Read the model definition and answer for the solid it produces. Units are mm, in the model's axes. Face numbers are marked on the shaded views. A direction names the side the tool comes from. Coordinates: 2 decimals unless noted, no trailing zeros. Write each loop counter-clockwise with the first axis right and the second up, starting at its lowest first coordinate (ties: lowest second). Pieces come first, ordered by that corner, then holes. Notation, with made-up numbers: (52, 11.5) -> (95, 11.5) arc R21 ccw to (95, 16.5) -> close; hole circle Ø9 at (33, 50). An arc over 180 degrees is marked (long way). Answer as a JSON object with one key per item and string values. Group by question number.
(1) Find section A-A (y = -11). Give the vertices of the cut face in (x, z).
(2) Straight lines are drawn through the part: L1, parallel to Y at x = 0, z = 14.4; L2, parallel to X at y = 1.65, z = -9.5; L3, parallel to Z at x = -1.75, y = -6.25. For each, find the intervals that lie inside material, in ascending order.
(3) Flat-ended cylindrical pins translate along their axes: P1, Ø4, axis at x = 0, z = -9.5, coming from the -Y side; P2, Ø4, axis at x = 0.5, y = -6, coming from the -Z side. Find the tip coordinate at first contact, or state that the pin passes through.
(4) Find section B-B (x = 0). Give the vertices of the cut face in (y, z).
(5) Which of the six approach directions +Z, -Z, +X, -X, +Y, -Y give full straight-line access (tool end or side, diameter ignored) to the marked faces 1 and 2?
(6) Find section C-C (z = -9.5). Give the vertices of the cut face in (x, y), then the cut area to 3 significant figures.
(7) Find section D-D (y = 0.5). Give the vertices of the cut face in (x, z).
(8) For a pull along Y with two mould halves and no side action, classify the marked faces 3, 4 and 5 as +Y half, -Y half, draft (parallel to the pull), parting line (faces both ways), or undercut.
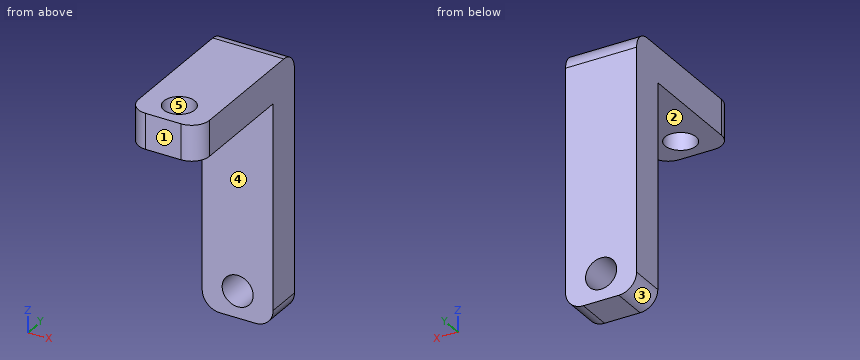
from build123d import *

# Parameters (mm, degrees)
ESQUISSE1_W        = 8
ESQUISSE1_H        = 25
ESQUISSE1_R        = 1.75
BOSS_EXTRU_1_DEPTH = 4
ESQUISSE2_W        = 8
ESQUISSE2_H        = 18
ESQUISSE2_R        = 1.75
BOSS_EXTRU_2_DEPTH = 4
CONG_1_R           = 2


with BuildPart() as part:
    # Esquisse1 → Boss.-Extru.1 (new body)
    with BuildSketch(Plane(origin=(0, 0, 0), x_dir=(1, 0, 0), z_dir=(0, 1, 0))):
        Rectangle(ESQUISSE1_W, ESQUISSE1_H)
        with Locations((0, 9.5)):
            Circle(ESQUISSE1_R, mode=Mode.SUBTRACT)
    extrude(amount=BOSS_EXTRU_1_DEPTH)

    # Esquisse2 → Boss.-Extru.2 (add)
    with BuildSketch(Plane.XY.offset(12.5)):
        with Locations((0, -5)):
            Rectangle(ESQUISSE2_W, ESQUISSE2_H)
        with Locations((0, -11)):
            Circle(ESQUISSE2_R, mode=Mode.SUBTRACT)
    extrude(amount=BOSS_EXTRU_2_DEPTH)

    # Congé1
    cong_1_edges = [part.edges().sort_by_distance(p)[0] for p in [
        (0, 4, 16.5),
        (-4, -14, 14.5),
        (4, -14, 14.5),
        (-4, 2, -12.5),
        (4, 2, -12.5),
    ]]
    fillet(cong_1_edges, radius=CONG_1_R)


solid = part.part
Results below:
{
 "1": {"outline": "(-4, 12.5) -> (-1.75, 12.5) -> (-1.75, 16.5) -> (-4, 16.5) -> close; (1.75, 12.5) -> (4, 12.5) -> (4, 16.5) -> (1.75, 16.5) -> close"},
 "2": {"L1": "y = -14 to -12.75, -9.25 to 4", "L2": "x = -4 to -1.75, 1.75 to 4", "L3": "z = 12.5 to 16.5"},
 "3": {"P1": "stops at y = 0", "P2": "stops at z = 12.5"},
 "4": {"outline": "(-14, 12.5) -> (-12.75, 12.5) -> (-12.75, 16.5) -> (-14, 16.5) -> close; (-9.25, 12.5) -> (0, 12.5) -> (0, -7.75) -> (4, -7.75) -> (4, 14.5) arc R2 ccw to (2, 16.5) -> (-9.25, 16.5) -> close; (0, -12.5) -> (4, -12.5) -> (4, -11.25) -> (0, -11.25) -> close"},
 "5": {"face 1": "+Z, -Z, +X, -X, -Y", "face 2": "-Z, +X, -X, -Y"},
 "6": {"outline": "(-4, 0) -> (-1.75, 0) -> (-1.75, 4) -> (-4, 4) -> close; (1.75, 0) -> (4, 0) -> (4, 4) -> (1.75, 4) -> close", "area": "18.0 mm2"},
 "7": {"outline": "(-4, -10.5) arc R2 ccw to (-2, -12.5) -> (2, -12.5) arc R2 ccw to (4, -10.5) -> (4, 16.5) -> (-4, 16.5) -> close; hole circle Ø3.5 at (0, -9.5)"},
 "8": {"face 3": "draft", "face 4": "-Y half", "face 5": "undercut"}
}
